For this review, take the finished solid that the model builds, in its own axes (mm). Face numbers are marked on the shaded views. Coordinates: 2 decimals unless noted, no trailing zeros. Order: outer loops, then holes, each group sorted by start corner. A loop starts at its lowest first (then second) coordinate and runs counter-clockwise, first axis right, second up.
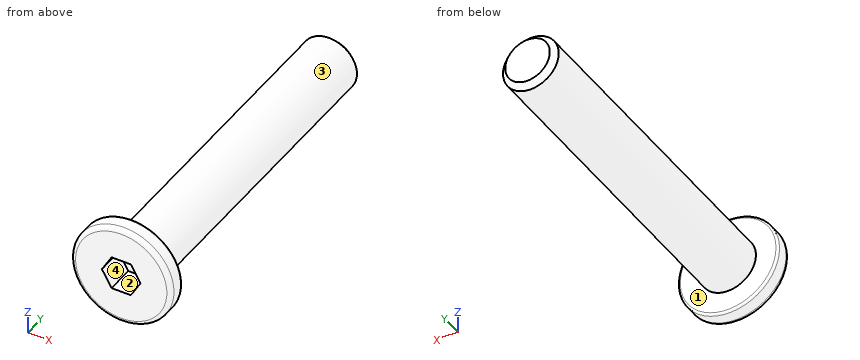
Autodesk Inventor part; units mm, degrees
ref_plane "YZ Plane" through (0, 0, 0) normal (1, 0, 0) x (0, 1, 0)
ref_plane "XZ Plane" through (0, 0, 0) normal (0, 1, 0) x (-1, 0, 0)
ref_plane "XY Plane" through (0, 0, 0) normal (0, 0, 1) x (1, 0, 0)
sketch "Boceto1" plane through (0, 0, 0) normal (0, 1, 0) x (-1, 0, 0)
  circle A0 centre (0, 0) radius 4.5
  dimension "d0" = 9
extrude "Extrusión1" add sketch "Boceto1" along normal blind 1.6
sketch "Boceto2" plane through (0, 1.6, 0) normal (0, 1, 0) x (1, 0, 0)
  circle A0 centre (0, 0) radius 2.5
  dimension "d3" = 5
extrude "Extrusión2" add sketch "Boceto2" along normal blind 30
fillet "Empalme1" radius 0.4 1 edges at (4.5, 0, 0)
fillet "Empalme2" radius 0.2 1 edges at (4.5, 1.6, 0)
sketch "Boceto3" plane through (0, 0, 0) normal (0, -1, 0) x (1, 0, 0)
  line L0 (-1.7321, 0) -> (-0.866, 1.5)
  line L1 (-0.866, 1.5) -> (0.866, 1.5)
  line L2 (0.866, 1.5) -> (1.7321, 0)
  line L3 (1.7321, 0) -> (0.866, -1.5)
  line L4 (0.866, -1.5) -> (-0.866, -1.5)
  line L5 (-0.866, -1.5) -> (-1.7321, 0)
  point P0 (0, 0)
  point P1 (0, 0)
  dimension "d8" = 3
extrude "Extrusión3" cut sketch "Boceto3" against normal blind 2.5
chamfer "Chaflán1" distance 0.5 angle 45 1 edges at (-2.5, 31.6, 0)
thread "Rosca2"
properties part number "Perno M5x8cabeza plana_" material "Hierro, gris"
1. Clearance check with flat-ended pins moving along their axes: pin 1 Ø1 at (x, y) = (-2.5, 23) entering from +Z; pin 2 Ø2 at (x, y) = (-2.5, 3.5) entering from -Z; pin 3 Ø4 at (y, z) = (4, 2.5) entering from +X. State where each tip first meets the part, or that it passes through.
Answer below:
pin 1: stops at z = 1.5
pin 2: stops at z = -2
pin 3: stops at x = 2.45
2. To check wall thickness, follow L1, parallel to Y at x = 1, z = -1; L2, parallel to Y at x = -1.25, z = -3.75; L3, parallel to X at y = 29, z = -1.5. State the ranges of each line that lie inside material, in increasing order.
Answer below:
L1: y = 2.5 to 31.6
L2: y = 0 to 1.6
L3: x = -2 to 2
3. Take a section at B-B, the plane y = 16. Give the boundary of the cut face in (x, z).
Answer below:
outline: circle Ø5 at (0, 0)
4. The part is to be moulded in two halves that separate along X. For the marked faces 1, 2, 3 and 4, say which applies: +X half, -X half, draft (parallel to the pull), parting line (faces both ways), or undercut.
Answer below:
face 1: draft
face 2: undercut
face 3: parting line
face 4: undercut
5. Take a section at A-A, the plane x = 0. Give the boundary of the cut face in (y, z), plus the area to 3 significant figures.
Answer below:
outline: (0, -4.1) arc R0.4 ccw to (0.4, -4.5) - (1.4, -4.5) arc R0.2 ccw to (1.6, -4.3) - (1.6, -2.5) - (31.1, -2.5) - (31.6, -2) - (31.6, 2) - (31.1, 2.5) - (1.6, 2.5) - (1.6, 4.3) arc R0.2 ccw to (1.4, 4.5) - (0.4, 4.5) arc R0.4 ccw to (0, 4.1) - (0, 1.5) - (2.5, 1.5) - (2.5, -1.5) - (0, -1.5) - close
area: 157 mm2
